Input: part model. Units: mm. Frame: model coordinates. Coordinates: 2 decimals unless noted, no trailing zeros. Loops run counter-clockwise (first coordinate to the right, second up) from the corner with the lowest first, then second, coordinate; pieces in that order, holes last.
(1) Section A-A, the plane z = 15. Return loops of the section in (x, y), then the cut area to 3 significant figures.
(2) Line query: L1, parallel to X at y = 0, z = 57.5; L2, parallel to Z at x = -38, y = -4; L3, parallel to X at y = 3.75, z = 15. Output: solid intervals per line, ascending.
(3) Contact query for flat-ended pins moving along their axis: P1, Ø1, axis at x = -25.5, y = 2.5, coming from the -Z side; P2, Ø2, axis at x = -76.23, y = 0, coming from the -Z side; P3, Ø2.5, axis at x = 81.63, y = 0, coming from the +Z side. Output: stop coordinate, or through.
```python
from build123d import *

# Parameters (mm, degrees)
SKETCH1_W                   = 210.475
SKETCH1_H                   = 9.525
BOSS_EXTRUDE1_DEPTH         = 63.9
SKETCH2_W                   = 40
SKETCH2_H                   = 20
CUT_EXTRUDE1_DEPTH          = 10.525
FILLET1_R                   = 12.7
TAP_DRILL_FOR_M4_TAP1_D     = 3.3
TAP_DRILL_FOR_M4_TAP1_DEPTH = 12.7
TAP_DRILL_FOR_M4_TAP1_TIP   = 0.991420021


with BuildPart() as part:
    # Sketch1 → Boss-Extrude1 (new body)
    with BuildSketch(Plane.XY):
        Rectangle(SKETCH1_W, SKETCH1_H)
    extrude(amount=BOSS_EXTRUDE1_DEPTH)

    # Sketch2 → Cut-Extrude1 (cut, through all)
    with BuildSketch(Plane(origin=(0, 4.7625, 0), x_dir=(1, 0, 0), z_dir=(0, 1, 0))):
        with Locations((-19.7625, -10)):
            Rectangle(SKETCH2_W, SKETCH2_H)
    extrude(amount=-CUT_EXTRUDE1_DEPTH, mode=Mode.SUBTRACT)

    # Fillet1
    fillet1_edges = [part.edges().sort_by_distance(p)[0] for p in [
        (-39.7625, 0, 20),
        (0.2375, 0, 20),
    ]]
    fillet(fillet1_edges, radius=FILLET1_R)

    # Tap Drill for M4 Tap1
    with Locations(Plane.XY.offset(63.9)):
        with Locations((-76.2285, 0), (2.6995, 0), (81.6285, 0)):
            Hole(TAP_DRILL_FOR_M4_TAP1_D / 2, depth=TAP_DRILL_FOR_M4_TAP1_DEPTH)
            with Locations((0, 0, -(TAP_DRILL_FOR_M4_TAP1_DEPTH + TAP_DRILL_FOR_M4_TAP1_TIP / 2))):  # 118° drill point
                Cone(0, TAP_DRILL_FOR_M4_TAP1_D / 2, TAP_DRILL_FOR_M4_TAP1_TIP, mode=Mode.SUBTRACT)


solid = part.part
```
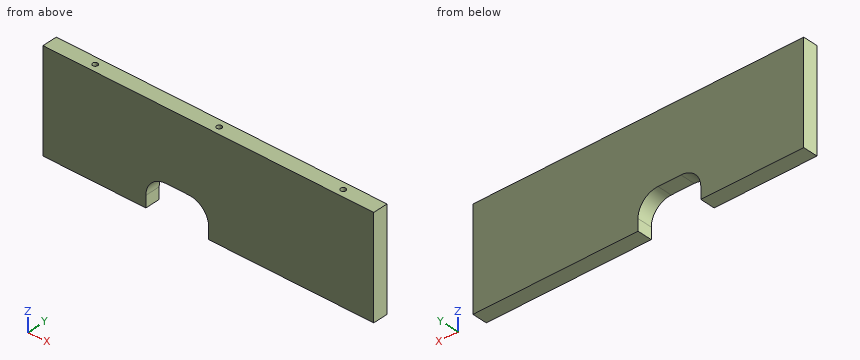
Report:
1. outline: (-105.24, -4.76) - (-37.16, -4.76) - (-37.16, 4.76) - (-105.24, 4.76) - close; (-2.36, -4.76) - (105.24, -4.76) - (105.24, 4.76) - (-2.36, 4.76) - close
1. area: 1,670 mm2
2. L1: x = -105.24 to -77.88, -74.58 to 1.05, 4.35 to 79.98, 83.28 to 105.24
2. L2: z = 13.75 to 63.9
2. L3: x = -105.24 to -37.16, -2.36 to 105.24
3. P1: stops at z = 20
3. P2: stops at z = 0
3. P3: stops at z = 50.96
